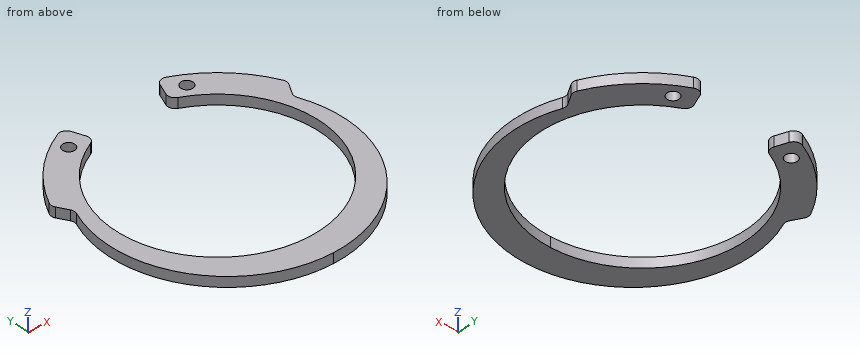
from build123d import *

# Parameters (mm, degrees)
SKETCH1_R           = 0.635
BOSS_EXTRUDE1_DEPTH = 0.5334
FILLET1_R           = 0.762


with BuildPart() as part:
    # Sketch1 → Boss-Extrude1 (new, symmetric)
    with BuildSketch(Plane.XY):
        with BuildLine():
            Line((0, -10.8712), (0, -13.7287))
            ThreePointArc((0, -13.7287), (10.539853689, -8.005916567), (11.480547007, 3.950414898))
            Line((11.480547007, 3.950414898), (12.490007611, 5.698851952))
            ThreePointArc((12.490007611, 5.698851952), (9.424661953, 9.982632457), (4.97184229, 12.796796003))
            Line((4.97184229, 12.796796003), (3.937, 10.13326307))
            ThreePointArc((3.937, 10.13326307), (10.685123278, -2.002780562), (0, -10.8712))
        make_face()
        with Locations((6.223, 10.609573083)):
            Circle(SKETCH1_R, mode=Mode.SUBTRACT)
    extrude(amount=BOSS_EXTRUDE1_DEPTH, both=True)

    # Fillet1
    fillet1_edges = [part.edges().sort_by_distance(p)[0] for p in [
        (12.490007611, 5.698851952, 0),
        (11.480547007, 3.950414898, 0),
        (3.937, 10.13326307, 0),
        (4.97184229, 12.796796003, 0),
    ]]
    fillet(fillet1_edges, radius=FILLET1_R)

    # Mirror1: part across plane


with BuildPart() as part_1:
    add(part.part)
    add(part.part.mirror(Plane(origin=(0, 0, 0), x_dir=(0, 0, 1), z_dir=(1, 0, 0))))


solid = part_1.part
Source: CAD feature listing. Evaluate the final solid. Frame: model axes, mm. Round coordinates to 2 decimals unless told otherwise and drop trailing zeros. Loops run counter-clockwise (first coordinate to the right, second up) from the corner with the lowest first, then second, coordinate; pieces in that order, holes last.
Q1. Ray query, line 1 (X direction, y = -1.5, z = -0.2); line 2 (Y direction, x = 7, z = -0.5); line 3 (X direction, y = -4.25, z = -0.15). Return the intervals inside material, ascending.
Q2. Section D-D, the plane x = 2.5. Return loops of the section in (y, z).
Q3. Section C-C, the plane z = 0.35. Return loops of the section in (x, y) (1 decimal), plus the area to 3 significant figures.
Q4. First-contact query: P1, Ø4, axis at x = 7, y = 3, coming from the -Z side; P2, Ø1.7, axis at x = -6.22, y = 10.61, coming from the +Z side. Flat tips, straight axial feed; report the tip coordinate or a pass-through.
Q5. Section A-A, the plane x = 9.75. Return loops of the section in (y, z), plus the area to 3 significant figures.
Q6. Section B-B, the plane y = -3.25. Return loops of the section in (x, z).
Solutions:
1. line 1: x = -12.56 to -10.77, 10.77 to 12.56
1. line 2: y = -11.6 to -8.32, 8.32 to 11.81
1. line 3: x = -12.18 to -10.01, 10.01 to 12.18
2. outline: (-13.48, -0.53) - (-10.58, -0.53) - (-10.58, 0.53) - (-13.48, 0.53) - close
3. outline: (-12.3, 5.4) - (-11.7, 4.3) arc R0.8 cw to (-11.6, 3.6) arc R12.6 ccw (long way) to (11.6, 3.6) arc R0.8 cw to (11.7, 4.3) - (12.3, 5.4) arc R0.8 ccw to (12.3, 6.1) arc R13.7 ccw to (5.7, 12.5) arc R0.8 ccw to (4.7, 12.1) - (4.2, 10.8) arc R0.8 ccw to (4.6, 9.9) arc R10.9 cw (long way) to (-4.6, 9.9) arc R0.8 ccw to (-4.2, 10.8) - (-4.7, 12.1) arc R0.8 ccw to (-5.7, 12.5) arc R13.7 ccw to (-12.3, 6.1) arc R0.8 ccw to start; hole circle Ø1.3 at (-6.2, 10.6); hole circle Ø1.3 at (6.2, 10.6)
3. area: 159 mm2
4. P1: passes through
4. P2: stops at z = 0.53
5. outline: (-9.09, -0.53) - (-4.81, -0.53) - (-4.81, 0.53) - (-9.09, 0.53) - close; (4.81, -0.53) - (9.67, -0.53) - (9.67, 0.53) - (4.81, 0.53) - close
5. area: 9.75 mm2
6. outline: (-12.39, -0.53) - (-10.37, -0.53) - (-10.37, 0.53) - (-12.39, 0.53) - close; (10.37, -0.53) - (12.39, -0.53) - (12.39, 0.53) - (10.37, 0.53) - close
